Model file for the job. Use its own axes, mm. A direction names the side the tool comes from. Round coordinates to 2 decimals unless told otherwise and drop trailing zeros. Order: outer loops, then holes, each group sorted by start corner. A loop starts at its lowest first (then second) coordinate and runs counter-clockwise, first axis right, second up. Notation, with made-up numbers: (37, -29) - (50, -29) arc R14 ccw to (50, -18) - close; hole circle Ø4 at (59.5, 24). An arc over 180 degrees is marked (long way). Use one line per item in the form item = value.
from build123d import *

# Parameters (mm, degrees)
SKETCH1_R           = 1.6
BOSS_EXTRUDE1_DEPTH = 3
SKETCH2_W           = 10
SKETCH2_H           = 10
BOSS_EXTRUDE2_DEPTH = 42
CHAMFER1_SIZE       = 5
SKETCH3_R           = 2.1
CUT_EXTRUDE1_DEPTH  = 52
SKETCH4_R           = 2.65
CUT_EXTRUDE2_DEPTH  = 0.5
SKETCH5_W           = 3
SKETCH5_H           = 43
BOSS_EXTRUDE3_DEPTH = 75
SKETCH6_W           = 3
SKETCH6_H           = 3.9
BOSS_EXTRUDE4_DEPTH = 2
SKETCH7_W           = 3
SKETCH7_H           = 68.8
BOSS_EXTRUDE5_DEPTH = 5
SKETCH8_R           = 1.5
CUT_EXTRUDE3_DEPTH  = 5


with BuildPart() as part:
    # Sketch1 → Boss-Extrude1 (new body)
    with BuildSketch(Plane(origin=(0, 0, 0), x_dir=(1, 0, 0), z_dir=(0, 1, 0))):
        Polygon((-6.512396694, 9.685950413), (1.487603306, 9.685950413), (26.487603306, 9.685950413), (26.487603306, -40.314049587), (1.487603306, -40.314049587), (-6.512396694, -40.314049587), align=None)
        with Locations(Location((-1.962396694, -35.764049587, 0), (0, 0, 270))):
            Circle(SKETCH1_R, mode=Mode.SUBTRACT)
        with Locations(Location((-1.962396694, 5.135950413, 0), (0, 0, 270))):
            Circle(SKETCH1_R, mode=Mode.SUBTRACT)
    extrude(amount=BOSS_EXTRUDE1_DEPTH)

    # Sketch2 → Boss-Extrude2 (add)
    with BuildSketch(Plane(origin=(0, 3, 0), x_dir=(1, 0, 0), z_dir=(0, 1, 0))):
        with Locations((21.487603306, -35.314049587)):
            Rectangle(SKETCH2_W, SKETCH2_H)
        with Locations((21.487603306, 4.685950413)):
            Rectangle(SKETCH2_W, SKETCH2_H)
    extrude(amount=BOSS_EXTRUDE2_DEPTH)

    # Chamfer1
    chamfer1_edges = [part.edges().sort_by_distance(p)[0] for p in [
        (21.487603306, 3, 30.314049587),
        (16.487603306, 3, 35.314049587),
        (16.487603306, 3, -4.685950413),
        (21.487603306, 3, 0.314049587),
    ]]
    chamfer(chamfer1_edges, length=CHAMFER1_SIZE)

    # Sketch3 → Cut-Extrude1 (cut)
    with BuildSketch(Plane(origin=(0, 45, 0), x_dir=(1, 0, 0), z_dir=(0, 1, 0))):
        with Locations(Location((22.537603306, -36.364049587, 0), (0, 0, 270))):
            Circle(SKETCH3_R)
        with Locations(Location((22.537603306, 5.735950413, 0), (0, 0, 270))):
            Circle(SKETCH3_R)
    extrude(amount=-CUT_EXTRUDE1_DEPTH, mode=Mode.SUBTRACT)

    # Sketch4 → Cut-Extrude2 (cut)
    with BuildSketch(Plane(origin=(0, 45, 0), x_dir=(1, 0, 0), z_dir=(0, 1, 0))):
        with Locations(Location((22.537603306, -36.364049587, 0), (0, 0, 270))):
            Circle(SKETCH4_R)
        with Locations(Location((22.537603306, 5.735950413, 0), (0, 0, 270))):
            Circle(SKETCH4_R)
    cut_extrude2 = extrude(amount=-CUT_EXTRUDE2_DEPTH, mode=Mode.SUBTRACT)

    # Mirror1: Cut-Extrude2 across plane
    add(cut_extrude2.mirror(Plane(origin=(0, 22.5, 0), x_dir=(0, 0, 1), z_dir=(0, -1, 0))), mode=Mode.SUBTRACT)

    # Sketch5 → Boss-Extrude3 (add)
    with BuildSketch(Plane.XY.offset(40.314049587)):
        with Locations((24.987603306, 21.5)):
            Rectangle(SKETCH5_W, SKETCH5_H)
    extrude(amount=BOSS_EXTRUDE3_DEPTH)

    # Sketch6 → Boss-Extrude4 (add)
    with BuildSketch(Plane(origin=(0, 43, 0), x_dir=(1, 0, 0), z_dir=(0, 1, 0))):
        with Locations((24.987603306, -44.564049587)):
            Rectangle(SKETCH6_W, SKETCH6_H)
    extrude(amount=BOSS_EXTRUDE4_DEPTH)

    # Sketch7 → Boss-Extrude5 (add)
    with BuildSketch(Plane(origin=(0, 43, 0), x_dir=(1, 0, 0), z_dir=(0, 1, 0))):
        with Locations((24.987603306, -80.914049587)):
            Rectangle(SKETCH7_W, SKETCH7_H)
    extrude(amount=BOSS_EXTRUDE5_DEPTH)

    # Sketch8 → Cut-Extrude3 (cut)
    with BuildSketch(Plane.ZY.offset(-23.487603306)):
        with Locations(Location((52.414049587, 44.5, 0), (0, 0, 270))):
            Circle(SKETCH8_R)
    extrude(amount=-CUT_EXTRUDE3_DEPTH, mode=Mode.SUBTRACT)


solid = part.part
(1) Slice it at B-B on z = -1. Give the cut face in (x, y).
Report:
outline = (-6.51, 0) - (26.49, 0) - (26.49, 45) - (16.49, 45) - (16.49, 8) - (11.49, 3) - (-6.51, 3) - close
(2) Slice it at C-C on x = 15. Give the cut face in (y, z).
Report:
outline = (0, -9.69) - (6.51, -9.69) - (6.51, 1.8) - (3, 5.31) - (3, 25.31) - (6.51, 28.83) - (6.51, 40.31) - (0, 40.31) - close
(3) Slice it at D-D on z = 104. Give the cut face in (x, y).
Report:
outline = (23.49, 0) - (26.49, 0) - (26.49, 48) - (23.49, 48) - close
(4) Tool access for faces 1 (the face through (25, 44.5, 36)), 2 (the face through (20, 45, 34)), 3 (the face through (25, 0.5, 36)), 4 (the face through (21, 26, 0.314)): list every direction of +Z, -Z, +X, -X, +Y, -Y with a clear straight run to the whole face (end or side of a thin tool).
Report:
face_1 = +Y
face_2 = -Z, +X, -X, +Y
face_3 = -Y
face_4 = +X, -X, +Y
(5) Pull direction Z, two halves, no side cores. Call faces 5 (the face through (16.488, 26, 35)), 6 (the face through (21.52, 44.75, -3.29)), 7 (the face through (25, 46, 46.514)): released by +Z, released by -Z, zero draft, split by the parting line, or undercut.
Report:
face_5 = zero draft
face_6 = undercut
face_7 = released by -Z
(6) Probe probe 1 along Z at (x, y) = (-1, 2); probe 2 along X at (y, z) = (28.5, 46.5); probe 3 along Y at (x, z) = (-3.5, 21.5). List the from-to ranges inside material, lowest first. Write a range as [from, to].
Report:
probe_1 = [-9.69, -6.41], [-3.86, 34.49], [37.04, 40.31]
probe_2 = [23.49, 26.49]
probe_3 = [0, 3]
(7) Pin check, flat tips, straight feed: pin 1 (2.5 mm diameter, centred on x = 23, z = -4.5, fed in from +Y); pin 2 (4 mm diameter, centred on x = -1.96, z = -5.14, fed in from +Y); pin 3 (8 mm diameter, centred on y = 28.5, z = 81, fed in from -X); pin 4 (2.5 mm diameter, centred on x = 22, z = 36.5, fed in from -Y). Stop position of each tip, or through.
Report:
pin_1 = 44.5
pin_2 = 3
pin_3 = 23.49
pin_4 = through
(8) Slice it at A-A on y = 38. Give the cut face in (x, z).
Report:
outline = (16.49, -9.69) - (26.49, -9.69) - (26.49, 0.31) - (16.49, 0.31) - close; (16.49, 30.31) - (26.49, 30.31) - (26.49, 115.31) - (23.49, 115.31) - (23.49, 40.31) - (16.49, 40.31) - close; hole circle Ø4.2 at (22.54, -5.74); hole circle Ø4.2 at (22.54, 36.36)
